Job drawing, mm, ordinate dimensions from the low corner. One solid piece. A direction names the side the tool comes from. Give positions to 0.01 mm unless a question says otherwise; leave off trailing zeros. Write each loop counter-clockwise with the first axis right and the second up, starting at its lowest first coordinate (ties: lowest second). Pieces come first, ordered by that corner, then holes. Notation, with made-up numbers: M 36.25,-33 L 91.25,-33 A30 ccw 91.25,-8 Z; hole C -23,-34.75 d6. An arc over 180 degrees is marked long. Answer as CSV lines item,"result". Start each with the question number.
Item 1: Pin check, flat tips, straight feed: pin 1 (6 mm diameter, centred on y = 6.5, z = 6.5, fed in from +X); pin 2 (5.5 mm diameter, centred on x = 23.5, y = 23.5, fed in from -Z); pin 3 (6 mm diameter, centred on x = 7, z = 4.5, fed in from +Y); pin 4 (4 mm diameter, centred on y = 5, z = 4.5, fed in from -X). Stop position of each tip, or through.
Item 2: Wall check: L1, parallel to Y at x = 23.5, z = 13.25; L2, parallel to Z at x = 23.5, y = 31.05; L3, parallel to Z at x = 43.5, y = 23.5. Give the ranges that are in metal, low to high. Write a range as from..to.
Item 3: Band-saw the part on D-D, the plane z = 7.5. List the corners of the cut face in (x, y), then the cut area to 3 significant figures.
Item 4: Band-saw the part on C-C, the plane z = 1.75. List the corners of the cut face in (x, y).
Item 5: Two-plate mould, pull along X, no slides. Class the marked faces 1, 2 and 3: +X half, -X half, draft (parallel to the pull), parting line (faces both ways), or undercut.
Item 6: Band-saw the part on B-B, the plane x = 23.5. List the corners of the cut face in (y, z), then the cut area to 3 significant figures.
Item 7: Band-saw the part on A-A, the plane y = 23.5. List the corners of the cut face in (x, z), then the cut area to 3 significant figures.
Item 8: 3-axis set-ups, long thin cutter, end or side, ignore diameter. For the marked faces 4 and 5: which of +Z, -Z, +X, -X, +Y, -Y reach the whole face in a straight line?
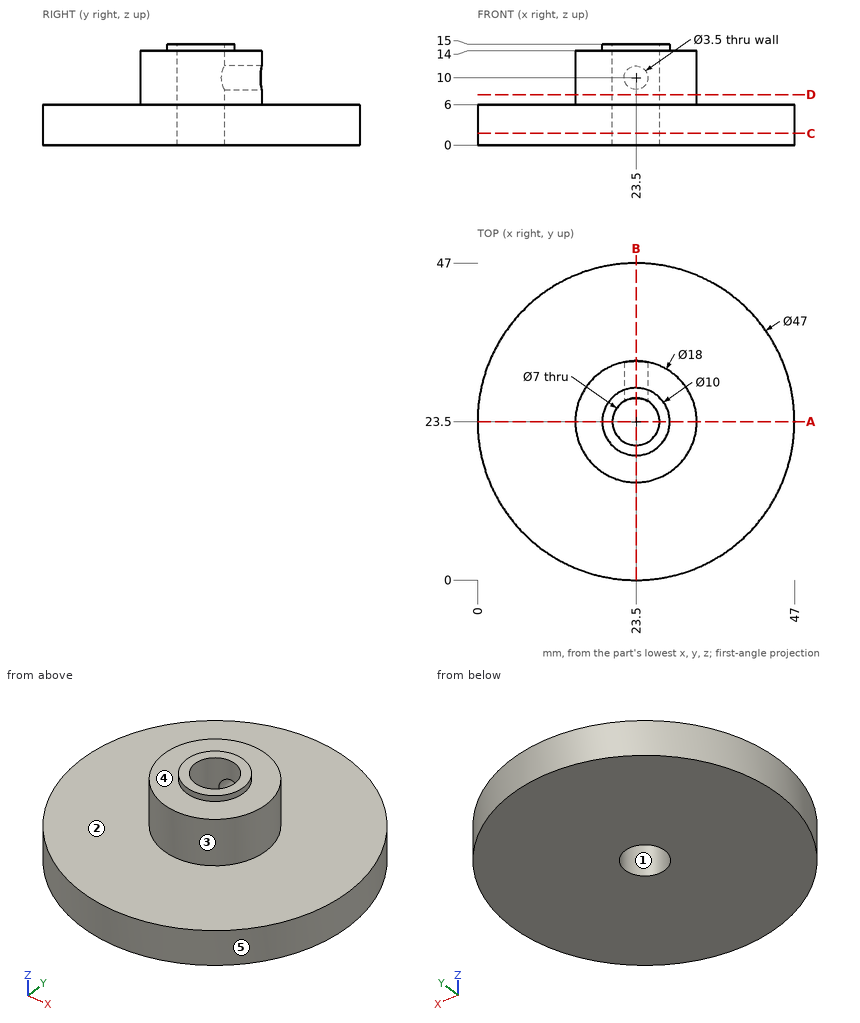
Output:
1,pin 1,"x = 42.34"
1,pin 2,"through"
1,pin 3,"y = 42.74"
1,pin 4,"x = 6.77"
2,L1,"14.5..20, 27..32.5"
2,L2,"0..8.25, 11.75..14"
2,L3,"0..6"
3,outline,"C 23.5,23.5 d18; hole C 23.5,23.5 d7"
3,area,"216 mm²"
4,outline,"C 23.5,23.5 d47; hole C 23.5,23.5 d7"
5,face 1,"undercut"
5,face 2,"draft"
5,face 3,"parting line"
6,outline,"M 0,0 L 20,0 L 20,15 L 18.5,15 L 18.5,14 L 14.5,14 L 14.5,6 L 0,6 Z; M 27,0 L 47,0 L 47,6 L 32.5,6 L 32.5,8.25 L 27,8.25 Z; M 27,11.75 L 32.5,11.75 L 32.5,14 L 28.5,14 L 28.5,15 L 27,15 Z"
6,area,"312 mm²"
7,outline,"M 0,0 L 20,0 L 20,15 L 18.5,15 L 18.5,14 L 14.5,14 L 14.5,6 L 0,6 Z; M 27,0 L 47,0 L 47,6 L 32.5,6 L 32.5,14 L 28.5,14 L 28.5,15 L 27,15 Z"
7,area,"331 mm²"
8,face 4,"+Z"
8,face 5,"+Z, -Z"
